```python
from build123d import *

# Parameters (mm, degrees)
PAD084_DEPTH    = 11
POCKET032_DEPTH = 10
SKETCH143_W     = 70.4
SKETCH143_H     = 30.4
POCKET033_DEPTH = 2.5
SKETCH144_R     = 5.5
POCKET034_DEPTH = 2.5


with BuildPart() as part:
    # Sketch141 → Pad084 (new body)
    with BuildSketch(Plane.XY):
        with BuildLine():
            ThreePointArc((-33, 18), (-36.535534, 16.535534), (-38, 13))
            Line((-38, 13), (-38, -13))
            ThreePointArc((-38, -13), (-36.535534, -16.535534), (-33, -18))
            Line((33, -18), (-33, -18))
            ThreePointArc((33, -18), (36.535534, -16.535534), (38, -13))
            Line((38, 13), (38, -13))
            ThreePointArc((38, 13), (36.535534, 16.535534), (33, 18))
            Line((-33, 18), (33, 18))
        make_face()
        with BuildLine():
            ThreePointArc((-33, 11), (-31.585786, 11.585786), (-31, 13))
            Line((-31, 13), (-5, 13))
            Line((-5, 13), (-5, -13))
            Line((-5, -13), (-31, -13))
            ThreePointArc((-31, -13), (-31.585786, -11.585786), (-33, -11))
            Line((-33, -11), (-33, 11))
        make_face(mode=Mode.SUBTRACT)
        with BuildLine():
            ThreePointArc((31, 13), (31.585786, 11.585786), (33, 11))
            Line((33, 11), (33, -11))
            ThreePointArc((33, -11), (31.585786, -11.585786), (31, -13))
            Line((31, -13), (5, -13))
            Line((5, 13), (5, -13))
            Line((5, 13), (31, 13))
        make_face(mode=Mode.SUBTRACT)
    extrude(amount=PAD084_DEPTH)

    # Sketch142 → Pocket032 (cut)
    with BuildSketch(Plane.XY.offset(12)):
        Polygon((-31, 18), (-31, 11), (-38, 11), (-38, -11), (-31, -11), (-31, -18), (31, -18), (31, -11), (38, -11), (38, 11), (31, 11), (31, 18), align=None)
    extrude(amount=-POCKET032_DEPTH, mode=Mode.SUBTRACT)

    # Sketch143 → Pocket033 (cut)
    with BuildSketch(Plane.XY.offset(6)):
        Rectangle(SKETCH143_W, SKETCH143_H)
    extrude(amount=POCKET033_DEPTH, mode=Mode.SUBTRACT)

    # Sketch144 → Pocket034 (cut)
    with BuildSketch(Plane.XY.offset(11)):
        with Locations((-33, -13)):
            Circle(SKETCH144_R)
        with Locations((33, -13)):
            Circle(SKETCH144_R)
    extrude(amount=-POCKET034_DEPTH, mode=Mode.SUBTRACT)

    # Cone008 → Cone008 (revolve, cut)
    with BuildSketch(Plane.XZ):
        Polygon((0, 0), (2, 0), (3, 2), (0, 2), align=None)
    revolve(axis=Axis((0, 0, 0), (0, 0, 1)), mode=Mode.SUBTRACT)


solid = part.part
```
Design review of the part built by this model. Coordinates are the model's own, in mm. A direction names the side the tool comes from. Round coordinates to 2 decimals unless told otherwise and drop trailing zeros. Write each loop counter-clockwise with the first axis right and the second up, starting at its lowest first coordinate (ties: lowest second). Pieces come first, ordered by that corner, then holes.
Item 1: We need section B-B on z = 5.25. Write out the cut boundary in (x, y).
Item 2: For faces 4 (the flat face through (-36, -11, 5)), 5 (the flat face through (35.2, 13, 7)), 6 (the flat face through (31, -16, 5)), list the 3-axis set-ups (+Z, -Z, +X, -X, +Y, -Y) from which the entire face can be reached by the end or side of a thin tool; tool diameter is ignored.
Item 3: We need section A-A on y = -7.5. Write out the cut boundary in (x, z).
Item 4: We need section C-C on x = 0. Write out the cut boundary in (y, z).
Item 5: For probe 1 along X at (y, z) = (6, 0.75); probe 2 along Y at (x, z) = (-7.5, 1); probe 3 along Z at (x, y) = (-8, 14.5), list the stretches that pass through material, from the lowest coordinate up.
Item 6: Clearance check with flat-ended pins moving along their axes: pin 1 Ø5.5 at (x, y) = (-36.5, -4) entering from +Z; pin 2 Ø3.5 at (x, y) = (35, -15) entering from +Z; pin 3 Ø6 at (y, z) = (-0.5, 5.5) entering from -X; pin 4 Ø2 at (x, y) = (-32.5, -13.5) entering from +Z. State where each tip first meets the part, or that it passes through.
Item 7: The part is to be moulded in two halves that separate along X. For faces 1 (the flat face through (-38, 0.2, 1.8)), 2 (the flat face through (18, -13, 1)), 3 (the flat face through (38, 0.2, 1.8)), say which applies: +X half, -X half, draft (parallel to the pull), parting line (faces both ways), or undercut.
Item 8: We need section D-D on y = 0. Write out the cut boundary in (x, z).
Returned:
1. outline: (-38, -13) arc R5 ccw to (-33, -18) - (-31, -18) - (-31, -13) arc R2 ccw to (-33, -11) - (-38, -11) - close; (-38, 11) - (-33, 11) arc R2 ccw to (-31, 13) - (-31, 18) - (-33, 18) arc R5 ccw to (-38, 13) - close; (31, -18) - (33, -18) arc R5 ccw to (38, -13) - (38, -11) - (33, -11) arc R2 ccw to (31, -13) - close; (31, 13) arc R2 ccw to (33, 11) - (38, 11) - (38, 13) arc R5 ccw to (33, 18) - (31, 18) - close
2. face 4: +Z, +X, -X
2. face 5: none
2. face 6: +Z, +Y, -Y
3. outline: (-38, 0) - (-33, 0) - (-33, 2) - (-38, 2) - close; (-5, 0) - (5, 0) - (5, 2) - (-5, 2) - close; (33, 0) - (38, 0) - (38, 2) - (33, 2) - close
4. outline: (-18, 0) - (-2, 0) - (-3, 2) - (-18, 2) - close; (2, 0) - (18, 0) - (18, 2) - (3, 2) - close
5. probe 1: x = -38 to -33, -5 to 5, 33 to 38
5. probe 2: y = -18 to -13, 13 to 18
5. probe 3: z = 0 to 2
6. pin 1: stops at z = 2
6. pin 2: stops at z = 8.5
6. pin 3: passes through
6. pin 4: stops at z = 6
7. face 1: -X half
7. face 2: undercut
7. face 3: +X half
8. outline: (-38, 0) - (-33, 0) - (-33, 2) - (-38, 2) - close; (-5, 0) - (-2, 0) - (-3, 2) - (-5, 2) - close; (2, 0) - (5, 0) - (5, 2) - (3, 2) - close; (33, 0) - (38, 0) - (38, 2) - (33, 2) - close
